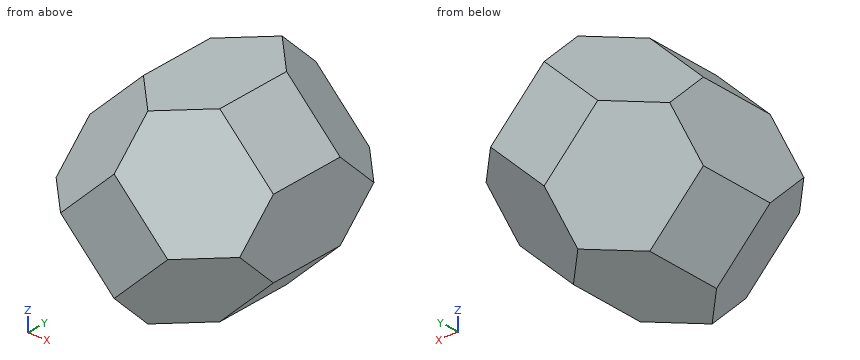
```python
from build123d import *

# Parameters (mm, degrees)
BOSS_EXTRUDE1_DEPTH  = 170
SKETCH2_W            = 70.7106781
SKETCH2_H            = 70
BOSS_EXTRUDE2_DEPTH  = 85
SKETCH3_W            = 70.208152808
SKETCH3_H            = 70
BOSS_EXTRUDE3_DEPTH  = 170.208153
BOSS_EXTRUDE7_DEPTH  = 140.710678
SKETCH5_W            = 70.208152808
SKETCH5_H            = 70
BOSS_EXTRUDE8_DEPTH  = 170.208153
BOSS_EXTRUDE9_DEPTH  = 40
BOSS_EXTRUDE10_DEPTH = 40
BOSS_EXTRUDE11_DEPTH = 40
BOSS_EXTRUDE14_DEPTH = 40
BOSS_EXTRUDE15_DEPTH = 40
BOSS_EXTRUDE17_DEPTH = 40
BOSS_EXTRUDE20_DEPTH = 40
BOSS_EXTRUDE21_DEPTH = 40
BOSS_EXTRUDE22_DEPTH = 40
BOSS_EXTRUDE24_DEPTH = 40


with BuildPart() as part:
    # Sketch1 → Boss-Extrude1 (new body)
    with BuildSketch(Plane.XY):
        Polygon((0, 0), (-35.355339059, 35.355339059), (-35.355339059, 105.355339059), (0, 140.710678119), (35.355339059, 105.355339059), (35.355339059, 35.355339059), align=None)
    extrude(amount=BOSS_EXTRUDE1_DEPTH)



with BuildPart() as body_2:
    # Sketch2 → Boss-Extrude2 (new, symmetric)
    with BuildSketch(Plane(origin=(0, 0, 0), x_dir=(0, 0, -1), z_dir=(1, 0, 0))):
        with Locations((-85, 70.355339059)):
            Rectangle(SKETCH2_W, SKETCH2_H)
        Polygon((-85, 140.710678109), (-120.35533905, 105.355339059), (-49.64466095, 105.355339059), align=None)
        Polygon((-49.64466095, 35.355339059), (-120.35533905, 35.355339059), (-85, 9e-09), align=None)
    extrude(amount=BOSS_EXTRUDE2_DEPTH, both=True)


with BuildPart() as part_1:
    add(part.part)

    add(body_2.part)  # Boss-Extrude3 merges body 2
    # Sketch3 → Boss-Extrude3 (add)
    with BuildSketch(Plane(origin=(17.677669533, 0, -17.67766953), x_dir=(-0.7071067811201199, 0, -0.7071067812529752), z_dir=(0.7071067812529752, 0, -0.7071067811201199))):
        with Locations((-60.104076402, 70.355339059)):
            Rectangle(SKETCH3_W, SKETCH3_H)
    extrude(amount=-BOSS_EXTRUDE3_DEPTH)

    # Sketch4 → Boss-Extrude7 (add)
    with BuildSketch(Plane(origin=(0, 140.710678119, 0), x_dir=(1, 0, 0), z_dir=(0, 1, 0))):
        Polygon((0, -35.355339059), (-49.64466095, -85.000000019), (0, -134.644660959), (49.64466095, -85), align=None)
    extrude(amount=-BOSS_EXTRUDE7_DEPTH)

    # Sketch5 → Boss-Extrude8 (add)
    with BuildSketch(Plane(origin=(-17.677669533, 0, -17.67766953), x_dir=(-0.7071067811201204, 0, 0.7071067812529747), z_dir=(-0.7071067812529747, 0, -0.7071067811201204))):
        with Locations((60.104076402, 70.355339059)):
            Rectangle(SKETCH5_W, SKETCH5_H)
    extrude(amount=-BOSS_EXTRUDE8_DEPTH)

    # Sketch7 → Boss-Extrude9 (add)
    with BuildSketch(Plane(origin=(0, 0, 0), x_dir=(0.8164965809277276, -0.4082482904638617, -0.4082482904638614), z_dir=(0.5773502691896236, 0.577350269189627, 0.5773502691896267))):
        Polygon((-104.103314072, -10.104076407), (-104.103314072, -60.104076394), (-60.802043892, -85.104076383), (-9e-09, -49.999999976), (0, 0), (-43.301270189, 25), align=None)
    extrude(amount=BOSS_EXTRUDE9_DEPTH)

    # Sketch8 → Boss-Extrude10 (add)
    with BuildSketch(Plane(origin=(0, 0, 0), x_dir=(-0.8164965809277275, -0.4082482904638613, -0.4082482904638619), z_dir=(0.5773502691896238, -0.5773502691896264, -0.5773502691896273))):
        Polygon((0, 0), (-104.103314072, -60.104076394), (-104.103314072, -10.104076407), (-43.301270189, 25), align=None)
        Polygon((0, 0), (5e-09, -50), (-60.802043877, -85.104076407), (-104.103314072, -60.104076394), align=None)
    extrude(amount=-BOSS_EXTRUDE10_DEPTH)

    # Sketch9 → Boss-Extrude11 (add)
    with BuildSketch(Plane(origin=(-8e-09, -35.355339028, -1e-08), x_dir=(-1.0, 2.324833960682746e-10, 0), z_dir=(-2.324833960682746e-10, -1.0, -2.9511459186104094e-10))):
        Polygon((-49.644660948, -85.000000014), (-1e-09, -35.355339056), (49.644660943, -85.000000003), (-1.9e-08, -134.644660946), align=None)
    extrude(amount=-BOSS_EXTRUDE11_DEPTH)

    # Sketch11 → Boss-Extrude14 (add)
    with BuildSketch(Plane(origin=(-56.666666664, -56.666666664, 56.666666669), x_dir=(0.8164965809396947, -0.408248290433944, 0.4082482904698449), z_dir=(-0.5773502691726996, -0.577350269172703, 0.5773502692234747))):
        Polygon((-34.701104701, 110.104076387), (-34.701104696, 60.1040764), (69.40220938, 120.208152796), (26.100939191, 145.208152798), align=None)
        Polygon((69.402209374, 70.208152796), (8.600165476, 35.104076398), (-34.701104696, 60.1040764), (69.40220938, 120.208152796), align=None)
    extrude(amount=-BOSS_EXTRUDE14_DEPTH)

    # Sketch12 → Boss-Extrude15 (add)
    with BuildSketch(Plane(origin=(56.666666687, -56.666666659, 56.666666659), x_dir=(0.40824829049722544, -0.40824829029705206, -0.8164965809944503), z_dir=(0.5773502693783509, -0.5773502690952631, 0.5773502690952634))):
        Polygon((-78.00237487, 85.104076392), (-138.804418754, 50.000000005), (-138.804418765, 6e-09), (-95.503148581, -25.000000002), (-34.701104701, 10.104076381), (-34.701104696, 60.104076393), align=None)
    extrude(amount=-BOSS_EXTRUDE15_DEPTH)

    # Sketch14 → Boss-Extrude17 (add)
    with BuildSketch(Plane(origin=(103.57022604, 103.57022604, 103.57022604), x_dir=(-0.8164965809277273, 0.4082482904638616, 0.4082482904638622), z_dir=(-0.5773502691896242, -0.5773502691896262, -0.5773502691896271))):
        Polygon((22.743789099, 39.393398276), (126.847103171, -20.710678119), (83.545832973, -45.710678114), (22.743789091, -10.606601707), align=None)
        Polygon((126.847103156, 29.289321886), (66.045059265, 64.393398279), (22.743789099, 39.393398276), (126.847103171, -20.710678119), align=None)
    extrude(amount=BOSS_EXTRUDE17_DEPTH)

    # Sketch15 → Boss-Extrude20 (add)
    with BuildSketch(Plane(origin=(-103.570226036, 103.570226036, 103.570226036), x_dir=(0.8164965809277289, 0.4082482904638593, 0.4082482904638611), z_dir=(-0.5773502691896217, 0.5773502691896265, 0.5773502691896291))):
        Polygon((126.847103171, -20.710678119), (83.545832973, -45.710678114), (22.743789099, -10.606601711), (22.743789099, 39.393398276), align=None)
        Polygon((66.045059273, 64.393398274), (126.847103156, 29.289321886), (126.847103171, -20.710678119), (22.743789099, 39.393398276), align=None)
    extrude(amount=-BOSS_EXTRUDE20_DEPTH)

    # Sketch18 → Boss-Extrude21 (add)
    with BuildSketch(Plane(origin=(-6e-09, 176.066017148, -3.1e-08), x_dir=(1.0, 3.131573767451649e-11, 0), z_dir=(-3.131573767451649e-11, 1.0, -1.7761984508401238e-10))):
        Polygon((-3e-09, -134.64466096), (49.644660968, -85.000000023), (-49.644660947, -85.000000026), align=None)
        Polygon((-49.644660947, -85.000000026), (-3e-09, -35.355339093), (49.644660968, -85.000000023), align=None)
    extrude(amount=-BOSS_EXTRUDE21_DEPTH)

    # Sketch19 → Boss-Extrude22 (add)
    with BuildSketch(Plane(origin=(46.90355937, 46.90355937, -46.90355937), x_dir=(-0.8164965809277273, 0.4082482904638619, -0.4082482904638618), z_dir=(-0.5773502691896241, -0.577350269189627, 0.5773502691896263))):
        Polygon((14.143623603, -74.497474683), (-46.65842028, -109.601551091), (-46.65842028, -159.601551077), (-3.357150107, -184.601551069), (57.444893789, -149.497474668), (57.444893792, -99.497474683), align=None)
    extrude(amount=BOSS_EXTRUDE22_DEPTH)

    # Sketch21 → Boss-Extrude24 (add)
    with BuildSketch(Plane(origin=(-46.903559392, 46.903559378, -46.903559356), x_dir=(-0.4082482903558565, 0.40824829023639164, 0.816496581095465), z_dir=(-0.5773502693927096, 0.5773502692237606, -0.5773502689524072))):
        Polygon((161.548207823, 89.393398286), (100.746163943, 124.497474679), (57.44489378, 99.497474694), (57.444893784, 49.497474694), (118.246937674, 14.393398298), (161.54820785, 39.393398295), align=None)
    extrude(amount=-BOSS_EXTRUDE24_DEPTH)


solid = part_1.part
```
Design review of the part built by this model. Coordinates are the model's own, in mm. Give positions to 0.01 mm unless a question says otherwise; leave off trailing zeros. Loops run counter-clockwise (first coordinate to the right, second up) from the corner with the lowest first, then second, coordinate; pieces in that order, holes last. Notation, with made-up numbers: M 32,-12 L 67,-12 A20 cw 67,4 Z; hole C 12,68.25 d10. An arc over 180 degrees is marked long. Return JSON: item names as keys, results as strings. Group by question number.
Item 1: We need section C-C (y = -21.5). Give the boundary of the cut face in (x, z), and give its area (3 significant figures).
Item 2: For probe 1 along Y at (x, z) = (-48.5, 36); probe 2 along Z at (x, y) = (-69.5, 139); probe 3 along Y at (x, z) = (34.5, 67), list the stretches that pass through material, from the lowest coordinate up.
Item 3: Insertion check: pin 1 Ø1.5 at (x, y) = (-61, -10.5) entering from -Z; pin 2 Ø5 at (x, z) = (25, 115) entering from +Y; pin 3 Ø3 at (x, z) = (59.5, 90.5) entering from +Y. Each pin has a flat end and moves straight along its axis. Give the tip position at first contact, or say it passes through.
Item 4: We need section D-D (x = -72.5). Give the boundary of the cut face in (y, z), and give its area (3 significant figures).
Item 5: We need section B-B (x = -25). Give the boundary of the cut face in (y, z).
Item 6: We need section A-A (y = 86). Give the boundary of the cut face in (x, z).
Output:
{
 "1": {"outline": "M -63.5,85 L 0,21.5 L 63.5,85 L 0,148.5 Z", "area": "8,060 mm^2"},
 "2": {"probe 1": "y = 12.5 to 128.21", "probe 2": "z = 67.79 to 102.21", "probe 3": "y = -32.5 to 173.21"},
 "3": {"pin 1": "stops at z = 70.44", "pin 2": "stops at y = 174.25", "pin 3": "stops at y = 162.83"},
 "4": {"outline": "M -12.5,85 L 35.36,37.14 L 105.36,37.14 L 153.21,85 L 105.36,132.86 L 35.36,132.86 Z", "area": "11,300 mm^2"},
 "5": {"outline": "M -35.36,60.36 L 25,0 L 115.71,0 L 176.07,60.36 L 176.07,109.64 L 115.71,170 L 25,170 L -35.36,109.64 Z"},
 "6": {"outline": "M -85,49.64 L -35.36,0 L 35.36,0 L 85,49.64 L 85,120.36 L 35.36,170 L -35.36,170 L -85,120.36 Z"}
}
